Design review of the part built by this model. Coordinates are the model's own, in mm. Face numbers are marked on the shaded views. Give positions to 0.01 mm unless a question says otherwise; leave off trailing zeros. Write each loop counter-clockwise with the first axis right and the second up, starting at its lowest first coordinate (ties: lowest second). Pieces come first, ordered by that corner, then holes.
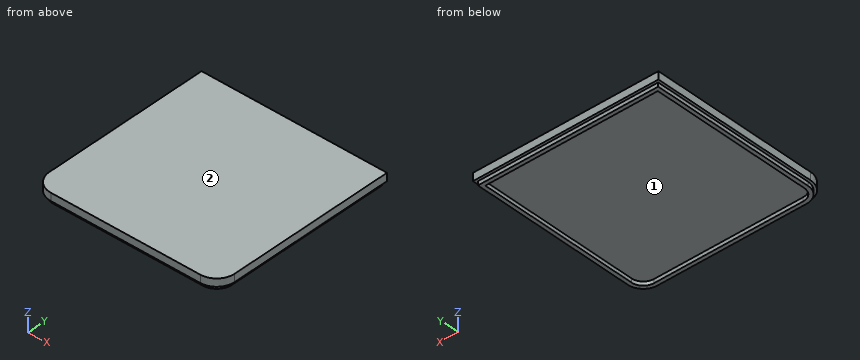
```python
from build123d import *

# Parameters (mm, degrees)
BOSS_EXTRUDE1_DEPTH = 6
BOSS_EXTRUDE2_DEPTH = 3


with BuildPart() as part:
    # Sketch1 → Boss-Extrude1 (new body)
    with BuildSketch(Plane.XY):
        with BuildLine():
            Line((-58, -72), (58, -72))
            ThreePointArc((58, -72), (67.899494937, -67.899494937), (72, -58))
            Line((72, -58), (72, 72))
            Line((72, 72), (-72, 72))
            Line((-72, 72), (-72, -58))
            ThreePointArc((-72, -58), (-67.899494937, -67.899494937), (-58, -72))
        make_face()
    extrude(amount=BOSS_EXTRUDE1_DEPTH)

    # Sketch2 → Boss-Extrude2 (add)
    with BuildSketch(Plane(origin=(0, 0, 0), x_dir=(-1, 0, 0), z_dir=(0, 0, -1))):
        with BuildLine():
            Line((-70, 70), (-70, -58))
            ThreePointArc((-70, -58), (-66.485281374, -66.485281374), (-58, -70))
            Line((-58, -70), (58, -70))
            ThreePointArc((58, -70), (66.485281374, -66.485281374), (70, -58))
            Line((70, -58), (70, 70))
            Line((70, 70), (-70, 70))
        make_face()
        with BuildLine():
            Line((-67, 67), (-67, -58))
            ThreePointArc((-67, -58), (-64.363961031, -64.363961031), (-58, -67))
            Line((-58, -67), (58, -67))
            ThreePointArc((58, -67), (64.363961031, -64.363961031), (67, -58))
            Line((67, -58), (67, 67))
            Line((67, 67), (-67, 67))
        make_face(mode=Mode.SUBTRACT)
    extrude(amount=BOSS_EXTRUDE2_DEPTH)


solid = part.part
```
(1) Consider section A-A, the plane x = 31. Give the boundary of the cut face in (y, z), then the cut area to 3 significant figures.
Resolved:
outline: (-72, 0) - (-70, 0) - (-70, -3) - (-67, -3) - (-67, 0) - (67, 0) - (67, -3) - (70, -3) - (70, 0) - (72, 0) - (72, 6) - (-72, 6) - close
area: 882 mm2
(2) Mouldability with a two-part tool opening along X and no side actions: class the marked faces 1 and 2 as pulls with the +X half, pulls with the -X half, needs draft (parallel to the pull), parting line crosses it, or undercut.
Resolved:
face 1: undercut
face 2: needs draft
(3) Clearance check with flat-ended pins moving along their axes: P1, Ø1.5, axis at y = -14, z = -1, coming from the +X side; P2, Ø3.5, axis at y = -25.5, z = -2, coming from the -X side; P3, Ø3.5, axis at x = -12.5, z = -2, coming from the +Y side. State where each tip first meets the part, or that it passes through.
Resolved:
P1: stops at x = 70
P2: stops at x = -70
P3: stops at y = 70
(4) To check wall thickness, follow L1, parallel to X at y = -6.5, z = -0.25; L2, parallel to Z at x = 29.5, y = 12. State the ranges of each line that lie inside material, in increasing order.
Resolved:
L1: x = -70 to -67, 67 to 70
L2: z = 0 to 6
